Geometry: final body of the model. Coordinates: model frame, mm. Face numbers are marked on the shaded views. A direction names the side the tool comes from. Give positions to 0.01 mm unless a question says otherwise; leave off trailing zeros. Loops run counter-clockwise (first coordinate to the right, second up) from the corner with the lowest first, then second, coordinate; pieces in that order, holes last. Notation, with made-up numbers: (11, 46.5) - (29, 46.5) arc R19 ccw to (29, 50.5) - close; hole circle Ø5 at (85.25, 72.25). An arc over 180 degrees is marked (long way). Use one line per item in the form item = value.
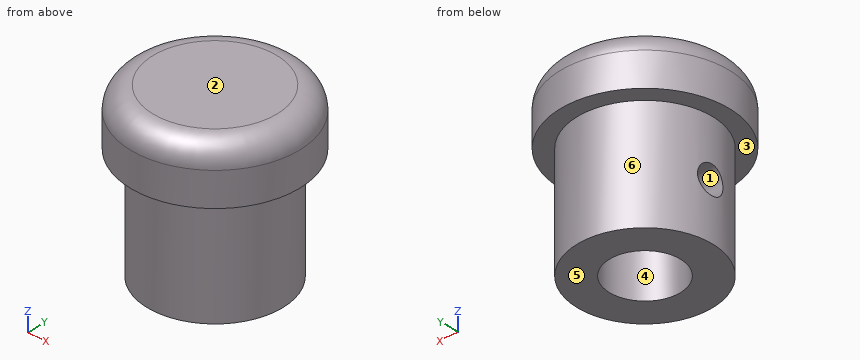
Autodesk Inventor part; units mm, degrees
ref_plane "YZ Plane" through (0, 0, 0) normal (1, 0, 0) x (0, 1, 0)
ref_plane "XZ Plane" through (0, 0, 0) normal (0, 1, 0) x (-1, 0, 0)
ref_plane "XY Plane" through (0, 0, 0) normal (0, 0, 1) x (1, 0, 0)
sketch "Sketch1" plane through (0, 0, 0) normal (0, 0, 1) x (1, 0, 0)
  circle A0 centre (0, 0) radius 3.15
  circle A1 centre (0, 0) radius 6
  dimension "d0" = 6.3
  dimension "d1" = 12
extrude "Extrusion1" add sketch "Sketch1" along normal blind 10
sketch "Sketch2" plane through (0, 0, 10) normal (0, 0, 1) x (1, 0, 0)
  circle A0 centre (0, 0) radius 7.5
  dimension "d4" = 15
extrude "Extrusion2" add sketch "Sketch2" along normal blind 5
fillet "Fillet1" radius 2 1 edges at (-7.5, 0, 15)
sketch "Sketch3" plane through (0, 0, 0) normal (1, 0, 0) x (0, 1, 0)
  line L0 (6, 0) -> (-6, 0)
  point P0 (0, 0)
  point P1 (0, 5)
  dimension "d8" = 5
hole "Hole1" at (0, 0, 5) direction (-1, 0, 0) diameter 2.5 end through all
properties part number "10-06-012 Joistic"
(1) Cut plane B-B (x = 0). Return the cut outline in (y, z).
Solution:
outline = (-7.5, 10) - (-6, 10) - (-6, 0) - (-3.15, 0) - (-3.15, 10) - (3.15, 10) - (3.15, 0) - (6, 0) - (6, 10) - (7.5, 10) - (7.5, 13) arc R2 ccw to (5.5, 15) - (-5.5, 15) arc R2 ccw to (-7.5, 13) - close
(2) Access query for the marked faces 1, 2 and 3. Directions: +Z, -Z, +X, -X, +Y, -Y. A direction counts if a zero-diameter tool reaches every point of the face in a straight line with its end or side. Return the directions, or none.
Solution:
face_1 = -X
face_2 = +Z, +X, -X, +Y, -Y
face_3 = -Z
(3) Cut plane A-A (y = 0). Return the cut outline in (x, z), plus the area to 3 significant figures.
Solution:
outline = (-7.5, 10) - (-6, 10) - (-6, 6.25) - (-3.15, 6.25) - (-3.15, 10) - (3.15, 10) - (3.15, 0) - (6, 0) - (6, 10) - (7.5, 10) - (7.5, 13) arc R2 ccw to (5.5, 15) - (-5.5, 15) arc R2 ccw to (-7.5, 13) - close; (-6, 0) - (-3.15, 0) - (-3.15, 3.75) - (-6, 3.75) - close
area = 123 mm2
(4) Material intervals for L1, parallel to X at y = 0, z = 7.5; L2, parallel to Z at x = -2, y = -1.25; L3, parallel to X at y = -1.5, z = 9.5, sorted ascending. Write a range as from..to.
Solution:
L1 = -6..-3.15, 3.15..6
L2 = 10..15
L3 = -5.81..-2.77, 2.77..5.81
(5) Pin query (flat end, axial travel): P1, Ø4, axis at x = 0, y = 0, coming from the -Z side; P2, Ø1, axis at y = -4, z = 2.5, coming from the -X side; P3, Ø2, axis at x = -0.5, z = 7, coming from the +Y side. Return the tip coordinate at first contact, or that it passes through.
Solution:
P1 = 10
P2 = -4.87
P3 = 6
(6) Cut plane C-C (z = 7.75). Return the cut outline in (x, y), plus the area to 3 significant figures.
Solution:
outline = circle Ø12 at (0, 0); hole circle Ø6.3 at (0, 0)
area = 81.9 mm2
(7) Pull-direction query (X, two-part tool) for the marked faces 4, 5 and 6; classes: released by +X, released by -X, zero draft, split by the parting line, or undercut.
Solution:
face_4 = undercut
face_5 = zero draft
face_6 = split by the parting line
(8) Cut plane D-D (z = 12). Return the cut outline in (x, y).
Solution:
outline = circle Ø15 at (0, 0)
